from build123d import *

# Parameters (mm, degrees)
SKETCH_2_R      = 2
SKETCH_2_R_2    = 1.5
EXTRUDE_2_DEPTH = 3


with BuildPart() as part:
    # 草图2 → 凸台-拉伸2 (new body)
    with BuildSketch(Plane(origin=(0, 0, 0), x_dir=(1, 0, 0), z_dir=(0, 1, 0))):
        with BuildLine():
            Line((-50, 0), (50, 0))
            Line((50, 0), (50, 10))
            Line((50, 10), (42, 10))
            ThreePointArc((42, 10), (39.878679656, 10.878679656), (39, 13))
            Line((39, 13), (39, 43.53))
            ThreePointArc((39, 43.53), (39.878679656, 45.651320344), (42, 46.53))
            Line((42, 46.53), (59, 46.53))
            ThreePointArc((59, 46.53), (61.121320344, 47.408679656), (62, 49.53))
            Line((62, 49.53), (62, 68.03))
            Line((62, 68.03), (73.21965962, 76.403723067))
            Line((73.21965962, 76.403723067), (82.431106141, 76.403723067))
            ThreePointArc((82.431106141, 76.403723067), (85.500981678, 77.839378281), (86.367215806, 81.115790975))
            Line((86.367215806, 81.115790975), (82.094808358, 104.732448965))
            ThreePointArc((82.094808358, 104.732448965), (80.723043479, 107.090256594), (78.158698693, 108.020381057))
            Line((78.158698693, 108.020381057), (73.5, 108.020381057))
            ThreePointArc((73.5, 108.020381057), (70.671572875, 106.848808182), (69.5, 104.020381057))
            Line((69.5, 104.020381057), (69.5, 96.092177826))
            ThreePointArc((69.5, 96.092177826), (69.363703305, 95.056901646), (68.964101615, 94.092177826))
            Line((68.964101615, 94.092177826), (64.309401077, 86.03))
            ThreePointArc((64.309401077, 86.03), (61.381197846, 83.10179677), (57.381197846, 82.03))
            Line((57.381197846, 82.03), (37.34, 82.03))
            ThreePointArc((37.34, 82.03), (32.34, 87.03), (27.34, 82.03))
            Line((27.34, 82.03), (-27.34, 82.03))
            ThreePointArc((-27.34, 82.03), (-32.34, 87.03), (-37.34, 82.03))
            Line((-37.34, 82.03), (-57.381197846, 82.03))
            ThreePointArc((-57.381197846, 82.03), (-61.381197846, 83.10179677), (-64.309401077, 86.03))
            Line((-64.309401077, 86.03), (-68.964101615, 94.092177826))
            ThreePointArc((-68.964101615, 94.092177826), (-69.363703305, 95.056901646), (-69.5, 96.092177826))
            Line((-69.5, 96.092177826), (-69.5, 104.020381057))
            ThreePointArc((-69.5, 104.020381057), (-70.671572875, 106.848808182), (-73.5, 108.020381057))
            Line((-73.5, 108.020381057), (-78.158698693, 108.020381057))
            ThreePointArc((-78.158698693, 108.020381057), (-80.723043479, 107.090256594), (-82.094808358, 104.732448965))
            Line((-82.094808358, 104.732448965), (-86.367215806, 81.115790975))
            ThreePointArc((-86.367215806, 81.115790975), (-85.500981678, 77.839378281), (-82.431106141, 76.403723067))
            Line((-82.431106141, 76.403723067), (-73.21965962, 76.403723067))
            Line((-73.21965962, 76.403723067), (-62, 68.03))
            Line((-62, 68.03), (-62, 49.53))
            ThreePointArc((-62, 49.53), (-61.121320344, 47.408679656), (-59, 46.53))
            Line((-59, 46.53), (-42.32, 46.53))
            ThreePointArc((-42.32, 46.53), (-40.198679656, 45.651320344), (-39.32, 43.53))
            Line((-39.32, 43.53), (-39.32, 13))
            ThreePointArc((-39.32, 13), (-40.198679656, 10.878679656), (-42.32, 10))
            Line((-42.32, 10), (-50.32, 10))
            Line((-50.32, 10), (-50.32, 0))
            Line((-50.32, 0), (-50, 0))
        make_face()
        with Locations(Location((40, 5, 0), (0, 0, 270))):
            Circle(SKETCH_2_R, mode=Mode.SUBTRACT)
        with Locations(Location((15, 5, 0), (0, 0, 270))):
            Circle(SKETCH_2_R, mode=Mode.SUBTRACT)
        with Locations(Location((57.84, 73.5, 0), (0, 0, 270))):
            Circle(SKETCH_2_R, mode=Mode.SUBTRACT)
        with Locations(Location((16.84, 14, 0), (0, 0, 270))):
            Circle(SKETCH_2_R, mode=Mode.SUBTRACT)
        with Locations(Location((78.158698693, 86.03, 0), (0, 0, 270))):
            Circle(SKETCH_2_R, mode=Mode.SUBTRACT)
        with Locations(Location((75.829349346, 99.527249228, 0), (0, 0, 270))):
            Circle(SKETCH_2_R, mode=Mode.SUBTRACT)
        with Locations(Location((-75.829349346, 99.527249228, 0), (0, 0, 90))):
            Circle(SKETCH_2_R, mode=Mode.SUBTRACT)
        with Locations(Location((-78.158698693, 86.03, 0), (0, 0, 90))):
            Circle(SKETCH_2_R, mode=Mode.SUBTRACT)
        with Locations(Location((-58.16, 73.5, 0), (0, 0, 90))):
            Circle(SKETCH_2_R, mode=Mode.SUBTRACT)
        with Locations(Location((-40.32, 5, 0), (0, 0, 90))):
            Circle(SKETCH_2_R, mode=Mode.SUBTRACT)
        with Locations(Location((-15.32, 5, 0), (0, 0, 90))):
            Circle(SKETCH_2_R, mode=Mode.SUBTRACT)
        with Locations(Location((-17.16, 14, 0), (0, 0, 270))):
            Circle(SKETCH_2_R, mode=Mode.SUBTRACT)
        with Locations(Location((32.34, 79, 0), (0, 0, 270))):
            Circle(SKETCH_2_R_2, mode=Mode.SUBTRACT)
        with BuildLine():
            Line((9, 25.5), (9, 36.5))
            ThreePointArc((9, 36.5), (12.5, 40), (16, 36.5))
            Line((16, 36.5), (16, 25.5))
            ThreePointArc((16, 25.5), (12.5, 22), (9, 25.5))
        make_face(mode=Mode.SUBTRACT)
        with BuildLine():
            Line((-9, 25.5), (-9, 36.5))
            ThreePointArc((-9, 36.5), (-12.5, 40), (-16, 36.5))
            Line((-16, 36.5), (-16, 25.5))
            ThreePointArc((-16, 25.5), (-12.5, 22), (-9, 25.5))
        make_face(mode=Mode.SUBTRACT)
        with BuildLine():
            Line((-25.272016313, 36.5), (-25.272016313, 25.5))
            ThreePointArc((-25.272016313, 25.5), (-28.772016313, 22), (-32.272016313, 25.5))
            Line((-32.272016313, 25.5), (-32.272016313, 36.5))
            ThreePointArc((-32.272016313, 36.5), (-28.772016313, 40), (-25.272016313, 36.5))
        make_face(mode=Mode.SUBTRACT)
        with BuildLine():
            Line((30.95778596, 36.5), (30.95778596, 25.5))
            ThreePointArc((30.95778596, 25.5), (27.45778596, 22), (23.95778596, 25.5))
            Line((23.95778596, 25.5), (23.95778596, 36.5))
            ThreePointArc((23.95778596, 36.5), (27.45778596, 40), (30.95778596, 36.5))
        make_face(mode=Mode.SUBTRACT)
        with BuildLine():
            Line((-34.733908774, 72.03), (-9.783415342, 59.322802138))
            ThreePointArc((-9.783415342, 59.322802138), (-9.263833402, 58.660781037), (-9.43365707, 57.836525462))
            Line((-9.43365707, 57.836525462), (-17.468690008, 46.988104116))
            ThreePointArc((-17.468690008, 46.988104116), (-18.279638575, 46.58331884), (-19.084539505, 47))
            Line((-19.084539505, 47), (-36, 70.555619208))
            ThreePointArc((-36, 70.555619208), (-35.946399549, 71.790395058), (-34.733908774, 72.03))
        make_face(mode=Mode.SUBTRACT)
        with BuildLine():
            Line((-22.298560337, 77.03), (-15.998560337, 77.03))
            ThreePointArc((-15.998560337, 77.03), (-15.376941046, 76.813319511), (-15.024707298, 76.257178913))
            Line((-15.024707298, 76.257178913), (-13.661633817, 70.41406068))
            ThreePointArc((-13.661633817, 70.41406068), (-13.87719951, 69.880514914), (-14.452198523, 69.903225894))
            Line((-14.452198523, 69.903225894), (-22.602198523, 76.13275467))
            ThreePointArc((-22.602198523, 76.13275467), (-22.77217551, 76.690276846), (-22.298560337, 77.03))
        make_face(mode=Mode.SUBTRACT)
        with BuildLine():
            Line((9.43365707, 57.836525462), (17.468690008, 46.988104116))
            ThreePointArc((17.468690008, 46.988104116), (18.279638575, 46.58331884), (19.084539505, 47))
            Line((19.084539505, 47), (36, 70.555619208))
            ThreePointArc((36, 70.555619208), (35.946399549, 71.790395058), (34.733908774, 72.03))
            Line((34.733908774, 72.03), (9.783415342, 59.322802138))
            ThreePointArc((9.783415342, 59.322802138), (9.263833402, 58.660781037), (9.43365707, 57.836525462))
        make_face(mode=Mode.SUBTRACT)
        with BuildLine():
            Line((14.452198523, 69.903225894), (22.602198523, 76.13275467))
            ThreePointArc((22.602198523, 76.13275467), (22.77217551, 76.690276846), (22.298560337, 77.03))
            Line((22.298560337, 77.03), (15.998560337, 77.03))
            ThreePointArc((15.998560337, 77.03), (15.376941046, 76.813319511), (15.024707298, 76.257178913))
            Line((15.024707298, 76.257178913), (13.661633817, 70.41406068))
            ThreePointArc((13.661633817, 70.41406068), (13.87719951, 69.880514914), (14.452198523, 69.903225894))
        make_face(mode=Mode.SUBTRACT)
        with BuildLine():
            Line((-3.013275549, 75.03), (-3.013275549, 70.43))
            ThreePointArc((-3.013275549, 70.43), (-2.77308317, 70.002799813), (-2.283275549, 69.986040542))
            Line((-2.283275549, 69.986040542), (2.156319027, 72.286040542))
            ThreePointArc((2.156319027, 72.286040542), (2.426319027, 72.73), (2.156319027, 73.173959458))
            Line((2.156319027, 73.173959458), (-2.283275549, 75.473959458))
            ThreePointArc((-2.283275549, 75.473959458), (-2.77308317, 75.457200187), (-3.013275549, 75.03))
        make_face(mode=Mode.SUBTRACT)
        with BuildLine():
            Line((3.013275549, 65.085839579), (3.013275549, 60.485839579))
            ThreePointArc((3.013275549, 60.485839579), (2.77308317, 60.058639392), (2.283275549, 60.041880121))
            Line((2.283275549, 60.041880121), (-2.156319027, 62.341880121))
            ThreePointArc((-2.156319027, 62.341880121), (-2.426319027, 62.785839579), (-2.156319027, 63.229799037))
            Line((-2.156319027, 63.229799037), (2.283275549, 65.529799037))
            ThreePointArc((2.283275549, 65.529799037), (2.77308317, 65.513039766), (3.013275549, 65.085839579))
        make_face(mode=Mode.SUBTRACT)
        with BuildLine():
            Line((-2.283275549, 49.986040542), (2.156319027, 52.286040542))
            ThreePointArc((2.156319027, 52.286040542), (2.426319027, 52.73), (2.156319027, 53.173959458))
            Line((2.156319027, 53.173959458), (-2.283275549, 55.473959458))
            ThreePointArc((-2.283275549, 55.473959458), (-2.77308317, 55.457200187), (-3.013275549, 55.03))
            Line((-3.013275549, 55.03), (-3.013275549, 50.43))
            ThreePointArc((-3.013275549, 50.43), (-2.77308317, 50.002799813), (-2.283275549, 49.986040542))
        make_face(mode=Mode.SUBTRACT)
    extrude(amount=EXTRUDE_2_DEPTH)


solid = part.part
Geometry: final body of the model. Coordinates: model frame, mm. A direction names the side the tool comes from. Round coordinates to 2 decimals unless told otherwise and drop trailing zeros. Write each loop counter-clockwise with the first axis right and the second up, starting at its lowest first coordinate (ties: lowest second). Pieces come first, ordered by that corner, then holes. Notation, with made-up numbers: M 50.5,-23 L 93.5,-23 A17 ccw 93.5,-8 Z; hole C 61,5 d2. An arc over 180 degrees is marked long. Write item = value, one per line.
Item 1: Section query C-C on y = 1.9. State how many separate pieces and enclosed holes the cut face has, then the cut area to 3 significant figures.
Findings:
separate_pieces = 1
enclosed_holes = 24
area = 8,290 mm^2
Item 2: Access query for faces 4 (the face through (12.4, 1.5, -40)), 5 (the face through (61.43, 1.48, -83.13)), 6 (the face through (67.531, 1.479, -72.158)). Directions: +Z, -Z, +X, -X, +Y, -Y. A direction counts if a zero-diameter tool reaches every point of the face in a straight line with its end or side. Return the directions, or none.
Findings:
face_4 = +Y, -Y
face_5 = -Z, +Y, -Y
face_6 = +Z, +X, +Y, -Y
Item 3: Section query A-A on z = -5. Return loops of the section in (x, y), then the cut area to 3 significant figures.
Findings:
outline = M -50.32,0 L -42.32,0 L -42.32,3 L -50.32,3 Z; M -38.32,0 L -17.32,0 L -17.32,3 L -38.32,3 Z; M -13.32,0 L 13,0 L 13,3 L -13.32,3 Z; M 17,0 L 38,0 L 38,3 L 17,3 Z; M 42,0 L 50,0 L 50,3 L 42,3 Z
area = 253 mm^2
Item 4: Pin query (flat end, axial travel): P1, Ø2.5, axis at x = -58.16, z = -73.5, coming from the -Y side; P2, Ø1.5, axis at x = -46.5, y = 2, coming from the -Z side; P3, Ø1.5, axis at y = 1, z = -29, coming from the -X side; P4, Ø0.9, axis at y = 1.5, z = -58.5, coming from the -X side. Return the tip coordinate at first contact, or that it passes through.
Findings:
P1 = through
P2 = -82.03
P3 = -39.32
P4 = -62
Item 5: Section query B-B on z = -29. Return loops of the section in (x, y).
Findings:
outline = M -39.32,0 L -32.27,0 L -32.27,3 L -39.32,3 Z; M -25.27,0 L -16,0 L -16,3 L -25.27,3 Z; M -9,0 L 9,0 L 9,3 L -9,3 Z; M 16,0 L 23.96,0 L 23.96,3 L 16,3 Z; M 30.96,0 L 39,0 L 39,3 L 30.96,3 Z
Item 6: Material intervals for line 1 along X through (y, z) = (2.15, -14); line 2 along X through (y, z) = (1.65, -5); line 3 along Z through (x, y) = (-58.5, 0.9), sorted ascending. Write a range as [from, to].
Findings:
line_1 = [-39.32, -19.16], [-15.16, 14.84], [18.84, 39]
line_2 = [-50.32, -42.32], [-38.32, -17.32], [-13.32, 13], [17, 38], [42, 50]
line_3 = [-82.11, -75.47], [-71.53, -46.53]
Item 7: Pull-direction query (X, two-part tool) for faces 1 (the face through (84.26, 1.48, -92.76)), 2 (the face through (-67.688, 1.479, -72.275)), 3 (the face through (17, 1, -5)); classes: pulls with the +X half, pulls with the -X half, needs draft (parallel to the pull), parting line crosses it, or undercut.
Findings:
face_1 = pulls with the +X half
face_2 = pulls with the -X half
face_3 = undercut
